```python
from build123d import *

# Parameters (mm, degrees)
F1_R     = 11
F1_R_2   = 9.8
F2_DEPTH = 3.5
F1_R_3   = 5.2
F1_R_4   = 4
F3_DEPTH = 3


with BuildPart() as f2:
    # F1 (on Top) → F2 (new body, symmetric)
    with BuildSketch(Plane.XY):
        Circle(F1_R)
        Circle(F1_R_2, mode=Mode.SUBTRACT)
    extrude(amount=F2_DEPTH, both=True)



with BuildPart() as f2b:
    # F1 (on Top) → F2, piece 2 (new body, symmetric)
    with BuildSketch(Plane.XY):
        Circle(F1_R_3)
        Circle(F1_R_4, mode=Mode.SUBTRACT)
    extrude(amount=F2_DEPTH, both=True)


with BuildPart() as f2_1:
    add(f2.part)

    add(f2b.part)  # F3 merges F2b
    # F1 (on Top) → F3 (join, symmetric)
    with BuildSketch(Plane.XY):
        Circle(F1_R_2)
        Circle(F1_R_3, mode=Mode.SUBTRACT)
    extrude(amount=F3_DEPTH, both=True)


solid = f2_1.part
```
Work out the finished part from the listing and answer in its coordinate system (mm). A direction names the side the tool comes from. Round coordinates to 2 decimals unless told otherwise and drop trailing zeros. Loops run counter-clockwise (first coordinate to the right, second up) from the corner with the lowest first, then second, coordinate; pieces in that order, holes last.
(1) The part is cut by section C-C, the plane x = 8.5. Give the vertices of the cut face in (y, z), and give its area (3 significant figures).
Computed values:
outline: (-6.98, -3.5) - (-4.88, -3.5) - (-4.88, -3) - (4.88, -3) - (4.88, -3.5) - (6.98, -3.5) - (6.98, 3.5) - (4.88, 3.5) - (4.88, 3) - (-4.88, 3) - (-4.88, 3.5) - (-6.98, 3.5) - close
area: 88.0 mm2
(2) The part is cut by section A-A, the plane x = 0. Give the vertices of the cut face in (y, z), and give its area (3 significant figures).
Computed values:
outline: (-11, -3.5) - (-9.8, -3.5) - (-9.8, -3) - (-5.2, -3) - (-5.2, -3.5) - (-4, -3.5) - (-4, 3.5) - (-5.2, 3.5) - (-5.2, 3) - (-9.8, 3) - (-9.8, 3.5) - (-11, 3.5) - close; (4, -3.5) - (5.2, -3.5) - (5.2, -3) - (9.8, -3) - (9.8, -3.5) - (11, -3.5) - (11, 3.5) - (9.8, 3.5) - (9.8, 3) - (5.2, 3) - (5.2, 3.5) - (4, 3.5) - close
area: 88.8 mm2
(3) The mould has two halves that part along X. Classify faces 4 (the cylindrical face through (-2.124, -9.567, 3.246)), 5 (the cylindrical face through (-0.867, -3.905, -0.049)), 6 (the cylindrical face through (-2.38, -10.74, 0.05)), 7 (the flat face through (-10, -1, -3.5)): pulls with the +X half, pulls with the -X half, needs draft (parallel to the pull), parting line crosses it, or undercut.
Computed values:
face 4: undercut
face 5: undercut
face 6: parting line crosses it
face 7: needs draft
(4) The part is cut by section D-D, the plane z = -2. Give the vertices of the cut face in (x, y).
Computed values:
outline: circle Ø22 at (0, 0); hole circle Ø8 at (0, 0)
(5) For faces 1 (the flat face through (3, -3, 3.5)), 2 (the cylindrical face through (-0.677, 5.156, -3.246)), 3 (the cylindrical face through (-0.677, 5.156, 3.254)), determine the directions among +Z, -Z, +X, -X, +Y, -Y from which every point of the face is accessible in a straight line to the end or side of a thin tool.
Computed values:
face 1: +Z, +X, -X, +Y, -Y
face 2: -Z
face 3: +Z
(6) Each of these flat-tipped pins is pushed along its axis until it touches: P1, Ø2, axis at x = 1.5, z = 0, coming from the -Y side; P2, Ø10, axis at x = -2, y = -2.5, coming from the -Z side; P3, Ø7, axis at x = 0, y = 0, coming from the +Z side; P4, Ø4, axis at y = -8, z = 1, coming from the +X side. Where does it stop, or does it pass through?
Computed values:
P1: stops at y = -10.99
P2: stops at z = -3.5
P3: passes through
P4: stops at x = 9.22
(7) Find the intervals of material crossed by L1, parallel to Y at x = 0, z = -3.3; L2, parallel to Y at x = 0, z = -1.5; L3, parallel to Z at x = -2.5, y = -8, in increasing order.
Computed values:
L1: y = -11 to -9.8, -5.2 to -4, 4 to 5.2, 9.8 to 11
L2: y = -11 to -4, 4 to 11
L3: z = -3 to 3
